Check sheet for the modelled part. Datum: model origin and axes. Units: mm. Round coordinates to 2 decimals unless told otherwise and drop trailing zeros. Write each loop counter-clockwise with the first axis right and the second up, starting at its lowest first coordinate (ties: lowest second). Pieces come first, ordered by that corner, then holes. Notation, with made-up numbers: M 13,87 L 21,87 A16 ccw 21,105 Z; hole C -30.75,43.5 d4. An arc over 180 degrees is marked long. Put each result on its own line as item: value.
```python
from build123d import *

# Parameters (mm, degrees)
F0_W      = 1270
F0_H      = 82.55
F1_DEPTH  = 12.7
F0_H_2    = 19.05
F1_FACE_W = 1270
F1_FACE_H = 82.55
F2_DEPTH  = 12.7
F3_SIZE2  = 50.8
F3_SIZE   = 12.7


with BuildPart() as f1:
    # F0 (on Top) → F1 (new body)
    with BuildSketch(Plane.XY):
        with Locations((378.9642523047, 18.4307628065)):
            Rectangle(F0_W, F0_H)
    extrude(amount=F1_DEPTH)

    # F0 (on Top) + F1_face (on face) → F2 (join)
    with BuildSketch(Plane.XY):
        with Locations((378.9642523047, 18.4307628065)):
            Rectangle(F0_W, F0_H)
        with Locations((378.9642523047, -32.3692371935)):
            Rectangle(F0_W, F0_H_2)
    with BuildSketch(Plane(origin=(378.9642523047, 18.4307628065, 12.7), x_dir=(1, 0, 0), z_dir=(0, 0, 1))):
        Rectangle(F1_FACE_W, F1_FACE_H)
    extrude(amount=F2_DEPTH)

    # F3
    f3_edges = [f1.edges().sort_by_distance(p)[0] for p in [
        (378.964252, 59.705763, 25.4),
    ]]
    f3_side = f1.faces().sort_by_distance((378.964252, 59.705763, 12.7))[0]
    chamfer(f3_edges, length=F3_SIZE, length2=F3_SIZE2, reference=f3_side)


solid = f1.part
```
1. Cross-section at A-A (x = 808). Enter the section's corners in (y, z).
Computed values:
outline: M -41.89,0 L 59.71,0 L 59.71,12.7 L 8.91,25.4 L -22.84,25.4 L -22.84,12.7 L -41.89,12.7 Z
2. Depth check by flat-ended pin: pin 1 Ø2 at (x, z) = (119, 17) entering from -Y. Enter the tip coordinate at first touch or a pass-through.
Computed values:
pin 1: stops at y = -22.84
3. Cross-section at C-C (z = 20.75). Enter the section's corners in (x, y).
Computed values:
outline: M -256.04,-22.84 L 1013.96,-22.84 L 1013.96,27.51 L -256.04,27.51 Z
4. Scan lines: probe 1 along Z at (x, y) = (717.5, 36.5); probe 2 along Z at (x, y) = (762.5, 16). Record each from-to range of solid material in increasing order.
Computed values:
probe 1: z = 0 to 18.5
probe 2: z = 0 to 23.63
5. Cross-section at B-B (y = 37.5). Enter the section's corners in (x, z), then the cut area to 3 significant figures.
Computed values:
outline: M -256.04,0 L 1013.96,0 L 1013.96,18.25 L -256.04,18.25 Z
area: 23,200 mm2
